Geometry check sheet. Reference: the model listing, model coordinates, mm. Coordinates: 2 decimals unless noted, no trailing zeros. Write each loop counter-clockwise with the first axis right and the second up, starting at its lowest first coordinate (ties: lowest second). Pieces come first, ordered by that corner, then holes. Notation, with made-up numbers: (-29.5, 83.25) -> (10.5, 83.25) arc R16 ccw to (10.5, 95.25) -> close; hole circle Ø1 at (6.25, -25.75). An arc over 180 degrees is marked (long way). Answer as CSV lines item,"result".
```python
from build123d import *

# Parameters (mm, degrees)
SKETCH1_W           = 59.5
SKETCH1_H           = 32.9
BOSS_EXTRUDE1_DEPTH = 16
FILLET1_R           = 5
SKETCH2_R           = 0.4
BOSS_EXTRUDE2_DEPTH = 12.7


with BuildPart() as part:
    # Sketch1 → Boss-Extrude1 (new body)
    with BuildSketch(Plane(origin=(0, 0, 0), x_dir=(1, 0, 0), z_dir=(0, 1, 0))):
        Rectangle(SKETCH1_W, SKETCH1_H)
    extrude(amount=BOSS_EXTRUDE1_DEPTH)

    # Fillet1
    fillet1_edges = [part.edges().sort_by_distance(p)[0] for p in [
        (0, 16, 16.45),
        (0, 16, -16.45),
    ]]
    fillet(fillet1_edges, radius=FILLET1_R)

    # Sketch2 → Boss-Extrude2 (add)
    with BuildSketch(Plane.XZ):
        with Locations(Location((27.165, 7.5, 0), (0, 0, 270))):
            Circle(SKETCH2_R)
        with Locations(Location((27.165, -7.5, 0), (0, 0, 270))):
            Circle(SKETCH2_R)
    extrude(amount=BOSS_EXTRUDE2_DEPTH)


solid = part.part
```
Item 1: Cross-section at B-B, the plane y = -10. Record the cut outline in (x, z) (3 decimals), plus the area to 3 significant figures.
Responses:
outline,"circle Ø0.8 at (27.165, -7.5); circle Ø0.8 at (27.165, 7.5)"
area,"1.01 mm2"
Item 2: Depth check by flat-ended pin: pin 1 Ø2 at (x, z) = (-7, 9) entering from -Y. Enter the tip coordinate at first touch or a pass-through.
Responses:
pin 1,"stops at y = 0"
Item 3: Thickness scan on probe 1 along Y at (x, z) = (20, -10.5); probe 2 along Z at (x, y) = (-5.5, 12); probe 3 along Y at (x, z) = (1.5, -13.5). Record the ranges inside material, lowest first.
Responses:
probe 1,"y = 0 to 16"
probe 2,"z = -16.35 to 16.35"
probe 3,"y = 0 to 15.56"
Item 4: Cross-section at C-C, the plane z = -10.5. Record the cut outline in (x, y), plus the area to 3 significant figures.
Responses:
outline,"(-29.75, 0) -> (29.75, 0) -> (29.75, 16) -> (-29.75, 16) -> close"
area,"952 mm2"
Item 5: Cross-section at A-A, the plane x = 23. Record the cut outline in (y, z), plus the area to 3 significant figures.
Responses:
outline,"(0, -16.45) -> (11, -16.45) arc R5 ccw to (16, -11.45) -> (16, 11.45) arc R5 ccw to (11, 16.45) -> (0, 16.45) -> close"
area,"516 mm2"
